Part model, mm, in its own coordinate system. A direction names the side the tool comes from. Give positions to 0.01 mm unless a question says otherwise; leave off trailing zeros. Order: outer loops, then holes, each group sorted by start corner. A loop starts at its lowest first (then second) coordinate and runs counter-clockwise, first axis right, second up. Notation, with made-up numbers: (-10.5, 56) - (44.5, 56) arc R19 ccw to (44.5, 63) - close; hole circle Ø6 at (11.25, 16.25). An arc over 180 degrees is marked (long way). One line per item, written item: value.
```python
from build123d import *

# Parameters (mm, degrees)
SKETCH1_W               = 28
SKETCH1_H               = 50
SKETCH1_R               = 5.5
BOSS_EXTRUDE1_DEPTH     = 6
SKETCH2_R               = 8.85
SKETCH2_R_2             = 7.85
BOSS_EXTRUDE2_DEPTH     = 9.5
SKETCH3_R               = 7.85
BOSS_EXTRUDE3_DEPTH     = 3.7
BOSS_EXTRUDE4_DEPTH     = 22
CHAMFER1_SIZE           = 7
BOSS_EXTRUDE5_DEPTH     = 2
BOSS_EXTRUDE6_DEPTH     = 2
BOSS_EXTRUDE7_DEPTH     = 9
CUT_EXTRUDE1_DEPTH      = 63.678335221
CUT_EXTRUDE1_DEPTH_BACK = 63.678335221
BOSS_EXTRUDE8_DEPTH     = 4
BOSS_EXTRUDE9_DEPTH     = 4
SKETCH12_R              = 6.85
BOSS_EXTRUDE10_DEPTH    = 4
SKETCH13_R              = 12
BOSS_EXTRUDE11_DEPTH    = 18
CHAMFER2_SIZE           = 2


with BuildPart() as part:
    # Sketch1 → Boss-Extrude1 (new body)
    with BuildSketch(Plane(origin=(0, 0, 0), x_dir=(0, 0, -1), z_dir=(1, 0, 0))):
        with Locations((14, -25)):
            Rectangle(SKETCH1_W, SKETCH1_H)
        with Locations((14, -12.7)):
            Circle(SKETCH1_R, mode=Mode.SUBTRACT)
    extrude(amount=BOSS_EXTRUDE1_DEPTH)

    # Sketch2 → Boss-Extrude2 (add)
    with BuildSketch(Plane(origin=(6, 0, 0), x_dir=(0, 0, -1), z_dir=(1, 0, 0))):
        with Locations((14, -12.7)):
            Circle(SKETCH2_R)
        with Locations((14, -12.7)):
            Circle(SKETCH2_R_2, mode=Mode.SUBTRACT)
    extrude(amount=BOSS_EXTRUDE2_DEPTH)

    # Sketch3 → Boss-Extrude3 (add)
    with BuildSketch(Plane(origin=(15.5, 0, 0), x_dir=(0, 0, -1), z_dir=(1, 0, 0))):
        with BuildLine():
            Line((2.15, -12.7), (2.15, -2.85))
            ThreePointArc((2.15, -2.85), (2.735786438, -1.435786438), (4.15, -0.85))
            Line((4.15, -0.85), (14, -0.85))
            ThreePointArc((14, -0.85), (22.379215357, -4.320784643), (25.85, -12.7))
            Line((25.85, -12.7), (25.85, -22.55))
            ThreePointArc((25.85, -22.55), (25.264213562, -23.964213562), (23.85, -24.55))
            Line((23.85, -24.55), (14, -24.55))
            ThreePointArc((14, -24.55), (11.74368498, -24.333208609), (9.569926867, -23.690766672))
            Line((9.569926867, -23.690766672), (3.402308332, -21.204770746))
            ThreePointArc((3.402308332, -21.204770746), (2.492383739, -20.46885486), (2.15, -19.34978903))
            Line((2.15, -19.34978903), (2.15, -12.7))
        make_face()
        with Locations((14, -12.7)):
            Circle(SKETCH3_R, mode=Mode.SUBTRACT)
    extrude(amount=BOSS_EXTRUDE3_DEPTH)

    # Sketch4 → Boss-Extrude4 (add)
    with BuildSketch(Plane(origin=(19.2, 0, 0), x_dir=(0, 0, -1), z_dir=(1, 0, 0))):
        with BuildLine():
            Line((21.85, -20.55), (6.15, -20.55))
            ThreePointArc((6.15, -20.55), (4.735786438, -19.964213562), (4.15, -18.55))
            Line((4.15, -18.55), (4.15, -13.55))
            Line((4.15, -13.55), (2.15, -13.55))
            Line((2.15, -13.55), (2.15, -19.34978903))
            ThreePointArc((2.15, -19.34978903), (2.252675107, -19.982369656), (2.55015825, -20.55))
            ThreePointArc((2.55015825, -20.55), (2.931431385, -20.935692725), (3.402308332, -21.204770746))
            Line((3.402308332, -21.204770746), (6.739747784, -22.55))
            Line((6.739747784, -22.55), (25.85, -22.55))
            Line((25.85, -22.55), (25.85, -20.55))
            Line((25.85, -20.55), (25.85, -13.55))
            Line((25.85, -13.55), (23.85, -13.55))
            Line((23.85, -13.55), (23.85, -18.55))
            ThreePointArc((23.85, -18.55), (23.264213562, -19.964213562), (21.85, -20.55))
        make_face()
    extrude(amount=BOSS_EXTRUDE4_DEPTH)

    # Chamfer1
    # the kernel refuses this chamfer: 7 mm, written as the material it takes off along each edge
    with BuildSketch(Plane(origin=(41.2, 4.451780916, -25.85), x_dir=(0.027495876610586112, 0, 0.9996219169112968), z_dir=(0, -1, 0))) as chamfer1_piece_1:
        Polygon((CHAMFER1_SIZE * 0.999621916911, CHAMFER1_SIZE * 0.0274958766106), (-CHAMFER1_SIZE * 0.0274958766106, CHAMFER1_SIZE * 0.999621916911), (0, 0), align=None)
    extrude(amount=45.003561832, mode=Mode.SUBTRACT)
    with BuildSketch(Plane(origin=(41.2, 4.451780916, -2.15), x_dir=(0.02749587661058612, 0, -0.9996219169112968), z_dir=(0, -1, 0))) as chamfer1_piece_2:
        Polygon((CHAMFER1_SIZE * 0.999621916911, -CHAMFER1_SIZE * 0.0274958766106), (-CHAMFER1_SIZE * 0.0274958766106, -CHAMFER1_SIZE * 0.999621916911), (0, 0), align=None)
    extrude(amount=41.803350861, mode=Mode.SUBTRACT)

    # Sketch6 → Boss-Extrude5 (add)
    with BuildSketch(Plane(origin=(16.025, 0, 16.025), x_dir=(0.7071067811865438, 0, -0.7071067811865512), z_dir=(0.7071067811865512, 0, 0.7071067811865438))):
        with BuildLine():
            Line((28.531758621, -13.55), (35.602826433, -13.55))
            Line((35.602826433, -13.55), (35.602826433, -20.55))
            Line((35.602826433, -20.55), (35.602826433, -22.55))
            Line((35.602826433, -22.55), (32.19421506, -22.55))
            Line((32.19421506, -22.55), (27.474362924, -21.204770746))
            add(Edge.make_bspline(
                [(25.703331496, -19.34978903), (25.703331496, -20.7), (27.474362924, -21.204770746)],
                knots=[0, 0, 0, 1.187644261, 1.187644261, 1.187644261], degree=2, weights=[1, 0.82880813, 1]))
            Line((25.703331496, -19.34978903), (25.703331496, -13.55))
            Line((25.703331496, -13.55), (28.531758621, -13.55))
        make_face()
    extrude(amount=BOSS_EXTRUDE5_DEPTH)

    # Sketch7 → Boss-Extrude6 (add)
    with BuildSketch(Plane(origin=(30.025, 0, -30.025), x_dir=(-0.7071067811865438, 0, -0.7071067811865512), z_dir=(0.7071067811865512, 0, -0.7071067811865438))):
        Polygon((-15.80383656, -20.55), (-15.80383656, -13.55), (-8.732768748, -13.55), (-5.904341623, -13.55), (-5.904341623, -22.55), (-15.80383656, -22.55), align=None)
    extrude(amount=BOSS_EXTRUDE6_DEPTH)

    # Sketch8 → Boss-Extrude7 (add)
    with BuildSketch(Plane(origin=(0, -13.55, 0), x_dir=(1, 0, 0), z_dir=(0, 1, 0))):
        Polygon((41.2, 18.85), (41.2, 9.15), (42.614213562, 7.735786438), (42.614213562, 20.264213562), align=None)
    extrude(amount=-BOSS_EXTRUDE7_DEPTH)

    # Sketch9 → Cut-Extrude1 (cut, two sides: drawn at the far end of the back side and taken through both)
    with BuildSketch(Plane(origin=(0, -13.55, 0), x_dir=(1, 0, 0), z_dir=(0, 1, 0)).offset(-CUT_EXTRUDE1_DEPTH_BACK)):
        Polygon((34.2, 2.15), (37.028427125, 2.15), (35.614213562, 0.735786438), align=None)
        Polygon((34.2, 25.85), (37.028427125, 25.85), (35.614213562, 27.264213562), align=None)
    extrude(amount=CUT_EXTRUDE1_DEPTH + CUT_EXTRUDE1_DEPTH_BACK, mode=Mode.SUBTRACT)

    # Sketch10 → Boss-Extrude8 (add)
    with BuildSketch(Plane(origin=(0, -20.55, 0), x_dir=(1, 0, 0), z_dir=(0, 1, 0))):
        with BuildLine():
            Line((34.7, 14), (34.7, 9))
            ThreePointArc((34.7, 9), (32.7, 7), (30.7, 9))
            Line((30.7, 9), (30.7, 14))
            ThreePointArc((30.7, 14), (32.7, 16), (34.7, 14))
        make_face()
    extrude(amount=BOSS_EXTRUDE8_DEPTH)

    # Sketch11 → Boss-Extrude9 (add)
    with BuildSketch(Plane(origin=(0, -16.55, 0), x_dir=(1, 0, 0), z_dir=(0, 1, 0))):
        with BuildLine():
            Line((18.505371288, 12.124502479), (32.005371288, 7.124502479))
            ThreePointArc((32.005371288, 7.124502479), (34.575497521, 8.305371288), (33.394628712, 10.875497521))
            Line((33.394628712, 10.875497521), (19.894628712, 15.875497521))
            ThreePointArc((19.894628712, 15.875497521), (17.324502479, 14.694628712), (18.505371288, 12.124502479))
        make_face()
    extrude(amount=BOSS_EXTRUDE9_DEPTH)

    # Sketch12 → Boss-Extrude10 (add)
    with BuildSketch(Plane(origin=(19.2, 0, 0), x_dir=(0, 0, -1), z_dir=(1, 0, 0))):
        with Locations((14, -12.7)):
            Circle(SKETCH12_R)
    extrude(amount=-BOSS_EXTRUDE10_DEPTH)

    # Sketch13 → Boss-Extrude11 (add)
    with BuildSketch(Plane.XZ.offset(22.55)):
        with Locations(Location((32.7, -14, 0), (0, 0, 142.769645669))):
            Circle(SKETCH13_R)
    extrude(amount=BOSS_EXTRUDE11_DEPTH)

    # Chamfer2
    chamfer2_edges = [part.edges().sort_by_distance(p)[0] for p in [
        (42.254513999, -40.55, -21.260252216),
    ]]
    chamfer(chamfer2_edges, length=CHAMFER2_SIZE)


solid = part.part
```
1) Cut at D-D, the plane y = -44. Give the cut face in (x, z).
Outcome:
outline: (0, -28) - (6, -28) - (6, 0) - (0, 0) - close
2) Cut at B-B, the plane x = 12.5. Give the cut face in (y, z).
Outcome:
outline: circle Ø17.7 at (-12.7, -14); hole circle Ø15.7 at (-12.7, -14)
3) Which spindle directions (+Z, -Z, +X, -X, +Y, -Y) get a long thin tool onto all of the face, cutting with end or side? Do faces 4 (the cylindrical face through (17.32, -23.95, -25.28)), 5 (the flat face through (30, -20.55, -14)), 6 (the cylindrical face through (17.32, -4.23, -22.29)), 7 (the flat face through (27, -12.55, -12)). Say none if no direction does.
Outcome:
face 4: -Z, -Y
face 5: none
face 6: -Z, +X, +Y
face 7: +Z, -Z, +X, +Y
4) Mould opens along X. For faces 1 (the flat face through (42.614, -18, -14)), 2 (the flat face through (30.7, -19, -11)), 3 (the flat face through (3, -25, 0)) say: released by +X, released by -X, zero draft, split by the parting line, or undercut.
Outcome:
face 1: released by +X
face 2: undercut
face 3: zero draft
5) Drill centre lines: line 1 along Y through (x, z) = (15.25, -14); line 2 along X through (y, z) = (-12, -20.25); line 3 along Y through (x, z) = (3.7, -14). Where is each one in solid material? Low to high. Write a range as from..to.
Outcome:
line 1: y = -21.55..-20.55, -19.55..-5.85, -4.85..-3.85
line 2: x = 0..6, 15.2..19.2
line 3: y = -50..-18.2, -7.2..0
6) Cut at A-A, the plane y = -6.5. Give the cut face in (x, z).
Outcome:
outline: (0, -28) - (6, -28) - (6, -20.32) - (15.5, -20.32) - (15.5, -24.1) - (19.2, -24.1) - (19.2, -18.81) - (6, -18.81) - (6, -9.19) - (19.2, -9.19) - (19.2, -2.15) - (15.5, -2.15) - (15.5, -7.68) - (6, -7.68) - (6, 0) - (0, 0) - close; (15.2, -16.91) - (19.2, -16.91) - (19.2, -11.09) - (15.2, -11.09) - close
7) Pin check, flat tips, straight feed: pin 1 (7 mm diameter, centred on y = -20, z = -13, fed in from +X); pin 2 (12 mm diameter, centred on x = 27.5, y = -10, fed in from -Z); pin 3 (3 mm diameter, centred on x = 21.5, z = -6, fed in from +Y); pin 4 (4 mm diameter, centred on x = 37.5, z = -18, fed in from +Y). Stop position of each tip, or through.
Outcome:
pin 1: stops at x = 44.7
pin 2: stops at z = -25.85
pin 3: stops at y = -19.68
pin 4: stops at y = -20.55
8) Cut at C-C, the plane x = 32.7. Give the cut face in (y, z), then the cut area to 3 significant figures.
Outcome:
outline: (-40.55, -24) - (-38.55, -26) - (-22.55, -26) - (-22.55, -25.85) - (-13.55, -25.85) - (-13.55, -23.85) - (-18.55, -23.85) arc R2 cw to (-20.55, -21.85) - (-20.55, -16) - (-16.55, -16) - (-16.55, -11.13) - (-12.55, -11.13) - (-12.55, -7) - (-20.55, -7) - (-20.55, -6.15) arc R2 cw to (-18.55, -4.15) - (-13.55, -4.15) - (-13.55, -2.15) - (-19.35, -2.15) arc R2 ccw to (-21.2, -3.4) - (-22.55, -6.74) - (-22.55, -2) - (-38.55, -2) - (-40.55, -4) - close
area: 553 mm^2
